from build123d import *

# Parameters (mm, degrees)
BOSS_EXTRUDE1_DEPTH   = 45
CUT_EXTRUDE1_START    = -5
CUT_EXTRUDE1_DEPTH    = 2
M4X0_7_TAPPED_HOLE1_D = 3.3
SKETCH5_R             = 7.5
BOSS_EXTRUDE2_DEPTH   = 45
SKETCH6_R             = 3.875
CUT_EXTRUDE2_DEPTH    = 46
CUT_EXTRUDE4_DEPTH    = 46


with BuildPart() as part:
    # Sketch1 → Boss-Extrude1 (new body)
    with BuildSketch(Plane.XY):
        with BuildLine():
            Line((-182.516015687, 162.517772537), (-172.5, 161.827012834))
            Line((-172.5, 161.827012834), (-172.5, 141.5))
            Line((-172.5, 141.5), (-162.5, 141.5))
            Line((-162.5, 141.5), (-162.5, 176.172987166))
            Line((-162.5, 176.172987166), (-181.483984313, 177.482227463))
            ThreePointArc((-181.483984313, 177.482227463), (-174.517772537, 169.483984313), (-182.516015687, 162.517772537))
        make_face()
    extrude(amount=BOSS_EXTRUDE1_DEPTH)

    # Sketch2 → Cut-Extrude1 (cut, symmetric)
    with BuildSketch(Plane(origin=(0, 0, 0), x_dir=(-1, 0, 0), z_dir=(0, 0, -1)).offset(CUT_EXTRUDE1_START)):
        with BuildLine():
            ThreePointArc((176.520836095, 177.139941379), (173.021327044, 169.380781175), (177.552867469, 162.175486453))
            ThreePointArc((177.552867469, 162.175486453), (177.834315887, 161.15284928), (176.811678714, 160.871400862))
            ThreePointArc((176.811678714, 160.871400862), (171.524881552, 169.277578038), (175.60764211, 178.329931609))
            ThreePointArc((175.60764211, 178.329931609), (176.659234217, 178.191533486), (176.520836095, 177.139941379))
        make_face()
    cut_extrude1 = extrude(amount=CUT_EXTRUDE1_DEPTH, both=True, mode=Mode.SUBTRACT)

    # Mirror1: Cut-Extrude1 across plane
    add(cut_extrude1.mirror(Plane(origin=(0, 0, 22.5), x_dir=(1, 0, 0), z_dir=(0, 0, -1))), mode=Mode.SUBTRACT)

    # M4x0.7 Tapped Hole1 (through all)
    with Locations(Plane.XY.offset(45)):
        with Locations((-167.5, 169), (-167.5, 146.5)):
            Hole(M4X0_7_TAPPED_HOLE1_D / 2)

    # Sketch5 → Boss-Extrude2 (add, through all)
    with BuildSketch(Plane.XY.offset(45)):
        with Locations((-182, 170)):
            Circle(SKETCH5_R)
    extrude(amount=-BOSS_EXTRUDE2_DEPTH)

    # Sketch6 → Cut-Extrude2 (cut, through all)
    with BuildSketch(Plane.XY.offset(45)):
        with Locations((-182, 170)):
            Circle(SKETCH6_R)
    extrude(amount=-CUT_EXTRUDE2_DEPTH, mode=Mode.SUBTRACT)

    # Sketch8 → Cut-Extrude4 (cut, through all)
    with BuildSketch(Plane.XY.offset(45)):
        with BuildLine():
            ThreePointArc((-178.929313469, 167.636420251), (-179.259961223, 167.259961223), (-179.636420251, 166.929313469))
            Line((-179.636420251, 166.929313469), (-178.818019485, 166.110912703))
            Line((-178.818019485, 166.110912703), (-178.110912703, 166.818019485))
            Line((-178.110912703, 166.818019485), (-178.929313469, 167.636420251))
        make_face()
        with BuildLine():
            Line((-182.5, 166.157393463), (-182.5, 165))
            Line((-182.5, 165), (-181.5, 165))
            Line((-181.5, 165), (-181.5, 166.157393463))
            ThreePointArc((-181.5, 166.157393463), (-182, 166.125), (-182.5, 166.157393463))
        make_face()
        with BuildLine():
            Line((-185.181980515, 166.110912703), (-184.363579749, 166.929313469))
            ThreePointArc((-184.363579749, 166.929313469), (-184.740038777, 167.259961223), (-185.070686531, 167.636420251))
            Line((-185.070686531, 167.636420251), (-185.889087297, 166.818019485))
            Line((-185.889087297, 166.818019485), (-185.181980515, 166.110912703))
        make_face()
        with BuildLine():
            Line((-187, 169.5), (-185.842606537, 169.5))
            ThreePointArc((-185.842606537, 169.5), (-185.875, 170), (-185.842606537, 170.5))
            Line((-185.842606537, 170.5), (-187, 170.5))
            Line((-187, 170.5), (-187, 169.5))
        make_face()
        with BuildLine():
            Line((-185.889087297, 173.181980515), (-185.070686531, 172.363579749))
            ThreePointArc((-185.070686531, 172.363579749), (-184.740038777, 172.740038777), (-184.363579749, 173.070686531))
            Line((-184.363579749, 173.070686531), (-185.181980515, 173.889087297))
            Line((-185.181980515, 173.889087297), (-185.889087297, 173.181980515))
        make_face()
        with BuildLine():
            Line((-182.5, 175), (-182.5, 173.842606537))
            ThreePointArc((-182.5, 173.842606537), (-182, 173.875), (-181.5, 173.842606537))
            Line((-181.5, 173.842606537), (-181.5, 175))
            Line((-181.5, 175), (-182.5, 175))
        make_face()
        with BuildLine():
            ThreePointArc((-179.636420251, 173.070686531), (-179.259961223, 172.740038777), (-178.929313469, 172.363579749))
            Line((-178.929313469, 172.363579749), (-178.110912703, 173.181980515))
            Line((-178.110912703, 173.181980515), (-178.818019485, 173.889087297))
            Line((-178.818019485, 173.889087297), (-179.636420251, 173.070686531))
        make_face()
        with BuildLine():
            ThreePointArc((-178.125, 170), (-178.133106846, 169.749475881), (-178.157393463, 169.5))
            Line((-178.157393463, 169.5), (-177, 169.5))
            Line((-177, 169.5), (-177, 170.5))
            Line((-177, 170.5), (-178.157393463, 170.5))
            ThreePointArc((-178.157393463, 170.5), (-178.133106846, 170.250524119), (-178.125, 170))
        make_face()
    extrude(amount=-CUT_EXTRUDE4_DEPTH, mode=Mode.SUBTRACT)


solid = part.part
Could you check a few things on this model? Use its own coordinates, in mm. A direction names the side the tool comes from. Coordinates: 2 decimals unless noted, no trailing zeros. Write each loop counter-clockwise with the first axis right and the second up, starting at its lowest first coordinate (ties: lowest second). Pieces come first, ordered by that corner, then holes. Notation, with made-up numbers: (-14.75, 17) - (5.25, 17) arc R20 ccw to (5.25, 23) - close; hole circle Ø8 at (16, -26). An arc over 180 degrees is marked (long way). Write item = value, one per line.
1) For faces 4 (the cylindrical face through (-173, 170, 5)), 5 (the flat face through (-182.5, 166, 23)), 6 (the flat face through (-173, 164, 45)), which set-ups out of +Z, -Z, +X, -X, +Y, -Y let a thin tool reach every point of the face, with its end or its side?
Result set:
face_4 = none
face_5 = +Z, -Z
face_6 = +Z, +X, -X, +Y, -Y
2) Suppose I cut it at B-B on x = -167.5. Please give me the cut outline in (y, z), plus the area to 3 significant figures.
Result set:
outline = (141.5, 0) - (144.85, 0) - (144.85, 45) - (141.5, 45) - close; (148.15, 0) - (167.35, 0) - (167.35, 45) - (148.15, 45) - close; (170.65, 0) - (176.52, 0) - (176.52, 45) - (170.65, 45) - close
area = 1,280 mm2
3) Suppose I cut it at C-C on z = 11.5. State how many separate pieces and enclosed holes the cut face has, plus the area to 3 significant figures.
Result set:
separate_pieces = 1
enclosed_holes = 3
area = 508 mm2
4) Please list where these lines run through material, in increasing order: line 1 (X direction, y = 146.5, z = 25.5); line 2 (Y direction, x = -167.5, z = 24.5); line 3 (X direction, y = 173.5, z = 28). Write a range as [from, to].
Result set:
line_1 = [-172.5, -169.15], [-165.85, -162.5]
line_2 = [141.5, 144.85], [148.15, 167.35], [170.65, 176.52]
line_3 = [-188.63, -185.57], [-184.79, -183.66], [-180.34, -179.21], [-178.43, -162.5]
5) We'd pull the mould along Y, two halves only. Please class faces 1 (the flat face through (-172.5, 152, 22)), 2 (the flat face through (-171.86, 176.82, 22.18)), 3 (the flat face through (-182.5, 174, 23)): +Y half, -Y half, draft (parallel to the pull), parting line (faces both ways), or undercut.
Result set:
face_1 = draft
face_2 = +Y half
face_3 = undercut
6) Will these pins go through, and if not, where does the flat tip stop? pin 1 Ø1 at (y, z) = (164, 12) entering from -X; pin 2 Ø4 at (y, z) = (152, 6.5) entering from -X; pin 3 Ø10 at (x, y) = (-169, 154.5) entering from -Z; pin 4 Ø4 at (x, z) = (-171, 24.5) entering from +Y.
Result set:
pin_1 = -187.1
pin_2 = -172.5
pin_3 = 0
pin_4 = 176.9
7) Suppose I cut it at A-A on y = 146.5. Please give me the cut outline in (x, z), plus the area to 4 significant figures.
Result set:
outline = (-172.5, 0) - (-169.15, 0) - (-169.15, 45) - (-172.5, 45) - close; (-165.85, 0) - (-162.5, 0) - (-162.5, 45) - (-165.85, 45) - close
area = 301.5 mm2
